from build123d import *

# Parameters (mm, degrees)
SKETCH1_R           = 3.375
SKETCH1_R_2         = 2.3749
BOSS_EXTRUDE1_DEPTH = 7.5
SKETCH2_R           = 1.49
CUT_EXTRUDE1_DEPTH  = 12.5


with BuildPart() as part:
    # Sketch1 → Boss-Extrude1 (new, symmetric)
    with BuildSketch(Plane.XY):
        Circle(SKETCH1_R)
        Circle(SKETCH1_R_2, mode=Mode.SUBTRACT)
    extrude(amount=BOSS_EXTRUDE1_DEPTH, both=True)

    # Sketch2 → Cut-Extrude1 (cut, symmetric)
    with BuildSketch(Plane(origin=(0, 0, 0), x_dir=(1, 0, 0), z_dir=(0, 1, 0))):
        with Locations(Location((0, -5, 0), (0, 0, 270))):
            Circle(SKETCH2_R)
    cut_extrude1 = extrude(amount=CUT_EXTRUDE1_DEPTH, both=True, mode=Mode.SUBTRACT)

    # Mirror1: Cut-Extrude1 across plane
    add(cut_extrude1.mirror(Plane.XY), mode=Mode.SUBTRACT)


solid = part.part
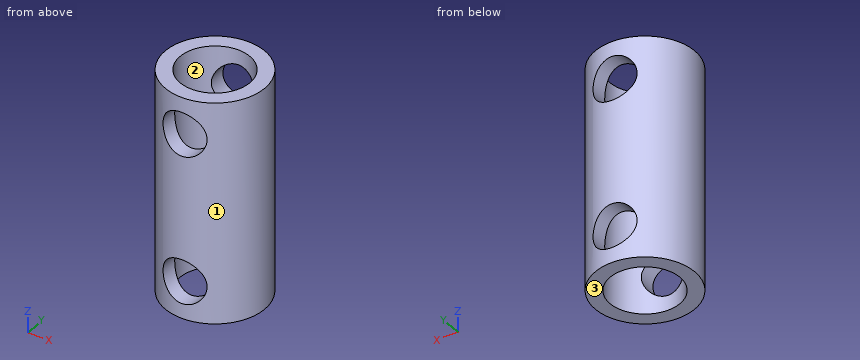
CAD build for the part. Positions are in the model's coordinates, mm. Face numbers are marked on the shaded views. Coordinates: 2 decimals unless noted, no trailing zeros. Write each loop counter-clockwise with the first axis right and the second up, starting at its lowest first coordinate (ties: lowest second). Pieces come first, ordered by that corner, then holes. Notation, with made-up numbers: (62, 9.5) - (94, 9.5) arc R32 ccw to (94, 43.5) - close; hole circle Ø11 at (85, 9.5). An arc over 180 degrees is marked (long way). Use a Markdown table: item, result. Add a question column.
Item 1: Mould opens along X. For the marked faces 1, 2 and 3 say: pulls with the +X half, pulls with the -X half, needs draft (parallel to the pull), parting line crosses it, or undercut.
Item 2: Flat gauge pins, fed straight in: pin 1 (4 mm diameter, centred on x = 0, z = 5, fed in from +Y) (3 decimals); pin 2 (1.5 mm diameter, centred on y = 1.5, z = 3, fed in from +X); pin 3 (1.8 mm diameter, centred on x = 0, z = -5, fed in from +Y); pin 4 (1 mm diameter, centred on y = 2, z = -4.5, fed in from -X). Where does each tip first touch, or does it go through?
Item 3: Band-saw the part on D-D, the plane z = -1.5. Give the cut face in (x, y) (3 decimals).
Item 4: Band-saw the part on A-A, the plane y = 0. Give the cut face in (x, z) (3 decimals), and give its area (3 significant figures).
Item 5: Drill centre lines: L1, parallel to Z at x = 0, y = -2.95; L2, parallel to Y at x = -2, z = 0; L3, parallel to Z at x = 1, y = -2.75. Where is each one in solid material? Low to high. Write a range as from..to.
Item 6: Band-saw the part on C-C, the plane z = -5.5. Give the cut face in (x, y) (3 decimals), and give its area (3 significant figures).
Item 7: Band-saw the part on B-B, the plane x = 0. Give the cut face in (y, z) (3 decimals), and give its area (3 significant figures).
Numbers:
| question | item | result |
|---|---|---|
| 1 | face 1 | parting line crosses it |
| 1 | face 2 | undercut |
| 1 | face 3 | needs draft |
| 2 | pin 1 | y = 3.375 |
| 2 | pin 2 | x = 3.29 |
| 2 | pin 3 | through |
| 2 | pin 4 | x = -3.02 |
| 3 | outline | circle Ø6.75 at (0, 0); hole circle Ø4.75 at (0, 0) |
| 4 | outline | (-3.375, -7.5) - (-2.375, -7.5) - (-2.375, 7.5) - (-3.375, 7.5) - close; (2.375, -7.5) - (3.375, -7.5) - (3.375, 7.5) - (2.375, 7.5) - close |
| 4 | area | 30.0 mm2 |
| 5 | L1 | -7.5..-6.49, -3.51..3.51, 6.49..7.5 |
| 5 | L2 | -2.72..-1.28, 1.28..2.72 |
| 5 | L3 | -7.5..-6.1, -3.9..3.9, 6.1..7.5 |
| 6 | outline | (-1.404, -3.069) - (-1.404, -1.916) arc R2.375 cw to (-1.404, 1.916) - (-1.404, 3.069) arc R3.375 ccw to start; (1.404, -3.069) arc R3.375 ccw to (1.404, 3.069) - (1.404, 1.916) arc R2.375 cw to (1.404, -1.916) - close |
| 6 | area | 12.2 mm2 |
| 7 | outline | (-3.375, -7.5) - (-2.375, -7.5) - (-2.375, -6.49) - (-3.375, -6.49) - close; (-3.375, -3.51) - (-2.375, -3.51) - (-2.375, 3.51) - (-3.375, 3.51) - close; (-3.375, 6.49) - (-2.375, 6.49) - (-2.375, 7.5) - (-3.375, 7.5) - close; (2.375, -7.5) - (3.375, -7.5) - (3.375, -6.49) - (2.375, -6.49) - close; (2.375, -3.51) - (3.375, -3.51) - (3.375, 3.51) - (2.375, 3.51) - close; (2.375, 6.49) - (3.375, 6.49) - (3.375, 7.5) - (2.375, 7.5) - close |
| 7 | area | 18.1 mm2 |
